Read the model definition and answer for the solid it produces. Units are mm, in the model's axes. Coordinates: 2 decimals unless noted, no trailing zeros. Write each loop counter-clockwise with the first axis right and the second up, starting at its lowest first coordinate (ties: lowest second). Pieces come first, ordered by that corner, then holes. Notation, with made-up numbers: M -11,12.5 L 23,12.5 A21 ccw 23,35.5 Z; hole C 63.25,77 d2. An arc over 180 degrees is marked long. Write item = value, one per line.
Autodesk Inventor part; units mm, degrees
ref_plane "Work Plane2" through (23.5818, 54.5446, 5) normal (0, 0.7488, -0.6628) x (-1, 0, 0)
ref_plane "YZ Plane" through (0, 0, 0) normal (1, 0, 0) x (0, 1, 0)
ref_plane "XZ Plane" through (0, 0, 0) normal (0, 1, 0) x (-1, 0, 0)
sketch "Sketch1" plane through (0, 0, 0) normal (0, 0, 1) x (1, 0, 0)
  line L0 (0, 0) -> (23.5818, 54.5446)
  line L1 (0, 0) -> (23.5818, -61.6289)
  line L2 (23.5818, -61.6289) -> (79.5818, -61.6289)
  line L3 (23.5818, 54.5446) -> (79.5818, 54.5446)
  line L4 (79.5818, 54.5446) -> (103.1637, 0)
  line L5 (103.1637, 0) -> (79.5818, -61.6289)
  circle A0 centre (5.7735, 0) radius 2.5
  circle A1 centre (97.3901, 0) radius 2.5
  dimension "d0" = 135.68
  dimension "d1" = 65.9865
  dimension "d2" = 59.424
  dimension "d3" = 56
  dimension "d4" = 65.9865
  dimension "d5" = 59.424
  dimension "d6" = 5
  dimension "d7" = 5
  dimension "d8" = 5.7735
  dimension "d9" = 5.7735
extrude "Extrusion1" add sketch "Sketch1" along normal blind 5
ref_plane "Work Plane2" through (23.5818, 54.5446, 5) normal (0, 0.7488, -0.6628) x (-1, 0, 0)
sketch "Sketch3" plane through (23.5818, 54.5446, 5) normal (0, 0.7488, -0.6628) x (-1, 0, 0)
  ellipse E0 centre (-73.8083, -39.894) end of major axis (-71.3083, -39.894) minor radius 1.6569
  ellipse E1 centre (17.8083, -39.894) end of major axis (20.3083, -39.894) minor radius 1.6569
  line L0 (23.5818, -39.894) -> (0, -3.7442)
  line L1 (0, -3.7442) -> (-56, -3.7442)
  line L2 (-56, -3.7442) -> (-79.5818, -39.894)
  line L3 (-79.5818, -39.894) -> (-56, -80.7389)
  line L4 (-56, -80.7389) -> (0, -80.7389)
  line L5 (0, -80.7389) -> (23.5818, -39.894)
  line L6 (-56, -3.7442) -> (-79.5818, -39.894)
  line L7 (-56, -3.7442) -> (-56, 0)
  line L8 (-79.5818, -36.1498) -> (-56, 0)
  line L9 (-79.5818, -39.894) -> (-79.5818, -36.1498)
  line L10 (0, -3.7442) -> (-56, -3.7442)
  line L11 (0, -3.7442) -> (0, 0)
  line L12 (-56, 0) -> (0, 0)
  line L13 (-56, -3.7442) -> (-56, 0)
  line L14 (0, 0) -> (23.5818, -36.1498)
  line L15 (23.5818, -39.894) -> (0, -3.7442)
  line L16 (23.5818, -39.894) -> (23.5818, -36.1498)
  line L17 (0, 0) -> (23.5818, -36.1498)
  line L18 (0, -3.7442) -> (0, 0)
extrude "Extrusion2" cut sketch "Sketch3" along normal through all contours E0 | E1 | L5 L4 L3 L2 L1 L0 | L0 L11 L14 L16 | L1 L7 L12 L11 | L2 L9 L8 L7
sketch "Sketch4" plane through (23.5818, 54.5446, 5) normal (0, 0.7488, -0.6628) x (1, 0, 0)
  line L0 (56, 0) -> (0, 0)
  line L1 (56, 0) -> (50.2265, -10)
  line L2 (50.2265, -10) -> (5.7735, -10)
  line L3 (5.7735, -10) -> (0, 0)
  line L4 (57.9132, 6.677) -> (56, 0)
  line L5 (79.5818, 36.1498) -> (56, 0)
  line L6 (79.5818, 39.894) -> (79.5818, 36.1498)
  line L7 (57.9132, 6.677) -> (79.5818, 39.894)
  line L8 (0, 0) -> (-1.9132, 6.677)
  line L9 (56, 0) -> (0, 0)
  line L10 (57.9132, 6.677) -> (56, 0)
  line L11 (-1.9132, 6.677) -> (57.9132, 6.677)
  line L12 (0, 0) -> (-1.9132, 6.677)
  line L13 (-23.5818, 39.894) -> (-1.9132, 6.677)
  line L14 (-23.5818, 39.894) -> (-23.5818, 36.1498)
  line L15 (0, 0) -> (-23.5818, 36.1498)
  dimension "d16" = 60
  dimension "d17" = 60
  dimension "d18" = 10
extrude "Extrusion3" add sketch "Sketch4" against normal blind 5 contours L1 L2 L3 L0 | L0 L8 L11 L4
sketch "Sketch5" plane through (23.5818, 54.5446, 5) normal (0, 0.7488, -0.6628) x (1, 0, 0)
  line L0 (0, 76.9948) -> (56, 76.9948)
  line L1 (56, 76.9948) -> (67.4601, 76.9948)
  line L2 (67.4601, 76.9948) -> (67.4601, 91.9948)
  line L3 (67.4601, 91.9948) -> (-7.5399, 91.9948)
  line L4 (0, 76.9948) -> (-7.5399, 76.9948)
  line L5 (-7.5399, 76.9948) -> (-7.5399, 91.9948)
  point P0 (-23.5818, 39.894)
  dimension "d21" = 15
  dimension "d22" = 75
extrude "Extrusion4" cut sketch "Sketch5" against normal through all
equation "\"d4\" = d1"
equation "\"d5\" = d2"
properties part number "TARM08" material "ABS Plastic"
Item 1: Find section D-D (y = 37.5). Determine the outline of the cut face in (x, z).
Worked answers:
outline = M 16.21,0 L 86.95,0 L 86.95,5 L 16.21,5 Z
Item 2: Consider line 1 along X through (y, z) = (-1, 4.5); line 2 along Z through (x, y) = (57, -31.5); line 3 along X through (y, z) = (13.5, 1). Determine where each line is inside the solid, lowest interval first. Write a range as from..to.
Worked answers:
line_1 = 0.38..3.48, 8.06..95.1, 99.68..102.78
line_2 = 0..5
line_3 = 5.84..97.33
Item 3: Flat-ended cylindrical pins translate along their axes: pin 1 (4 mm diameter, centred on x = 72.5, z = 9, fed in from +Y); pin 2 (6 mm diameter, centred on x = 87.5, y = 19, fed in from +Z). Find the tip coordinate at first contact, or state that the pin passes through.
Worked answers:
pin_1 = 59.86
pin_2 = 5
Item 4: Find section A-A (z = 3.5). Determine the outline of the cut face in (x, y), and give its area (3 significant figures).
Worked answers:
outline = M 0,0 L 22.93,-59.93 L 80.23,-59.93 L 103.16,0 L 80.16,53.22 L 23.01,53.22 Z; hole C 5.77,0 d5; hole C 97.39,0 d5
area = 9,030 mm²
Item 5: Find section C-C (y = -15). Determine the outline of the cut face in (x, z), and give its area (3 significant figures).
Worked answers:
outline = M 5.74,0 L 97.42,0 L 97.42,5 L 5.74,5 Z
area = 458 mm²
Item 6: For a pull along Y with two mould halves and no side action, classify faces 1 (the face through (51, -2, 0)), 2 (the face through (94.893, -0.11, 2.465)), 3 (the face through (8.16, -0.75, 2.46)), 4 (the face through (76.735, 55.966, 10.325)) as released by +Y, released by -Y, zero draft, split by the parting line, or undercut.
Worked answers:
face_1 = zero draft
face_2 = undercut
face_3 = undercut
face_4 = released by +Y
Item 7: Find section B-B (x = 63). Determine the outline of the cut face in (y, z), and give its area (3 significant figures).
Worked answers:
outline = M -61.62,5 L -55.97,0 L 50.12,0 L 61.17,12.49 L 57.43,15.8 L 47.87,5 Z
area = 617 mm²
